Source: CAD feature listing. Evaluate the final solid. Frame: model axes, mm. Face numbers are marked on the shaded views. Round coordinates to 2 decimals unless told otherwise and drop trailing zeros. Loops run counter-clockwise (first coordinate to the right, second up) from the corner with the lowest first, then second, coordinate; pieces in that order, holes last. Notation, with made-up numbers: M 9.5,-19.5 L 21.5,-19.5 A25 ccw 21.5,18.5 Z; hole C 3,-31 d9. An arc over 180 degrees is marked long. Answer as CSV lines item,"result". Start each with the question number.
```python
from build123d import *

# Parameters (mm, degrees)
F0_R     = 15
F1_DEPTH = 180
F2_R     = 12.25
F3_DEPTH = 180
F4_R     = 12.25
F5_DEPTH = 180


# Not quite as in the source:
# - the program builds the solid bodies; features that only make, move or delete a surface that nothing else refers to are left out


with BuildPart() as f1:
    # F0 (on Front) → F1 (new body)
    with BuildSketch(Plane.XZ):
        Circle(F0_R)
    extrude(amount=F1_DEPTH)

    # F2 (on Front) → F3 (cut)
    with BuildSketch(Plane.XZ):
        Circle(F2_R)
    extrude(amount=-F3_DEPTH, mode=Mode.SUBTRACT)

    # F4 (on Front) → F5 (cut)
    with BuildSketch(Plane.XZ):
        Circle(F4_R)
    extrude(amount=F5_DEPTH, mode=Mode.SUBTRACT)


solid = f1.part
```
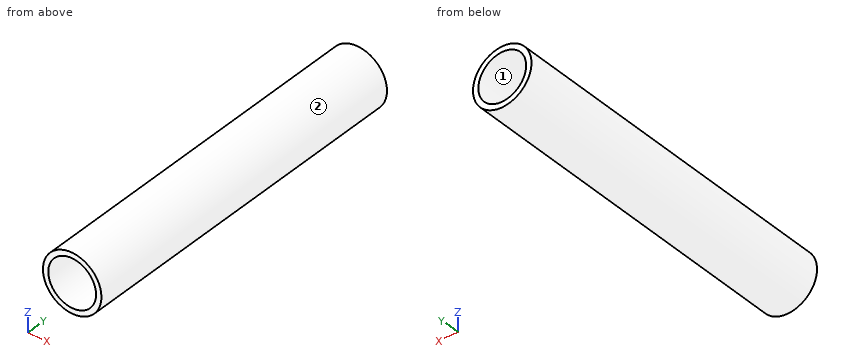
1) Ray query, line 1 along Z through (x, y) = (0, -47); line 2 along X through (y, z) = (-124, 0.75); line 3 along X through (y, z) = (-139, -7.5). Return the intervals inside material, ascending.
2) Section B-B, the plane x = 0. Return loops of the section in (y, z).
3) Section A-A, the plane z = 0. Return loops of the section in (x, y), and give its area (3 significant figures).
4) Mould query, pull axis Z, two halves, no side actions, for the marked faces 1 and 2. Classes: pulls with the +Z half, pulls with the -Z half, needs draft (parallel to the pull), parting line crosses it, or undercut.
5) Contact query for flat-ended pins moving along their axis: pin 1 Ø5 at (y, z) = (-108, -6) entering from -X; pin 2 Ø1 at (y, z) = (-84.5, 4) entering from +X; pin 3 Ø10 at (y, z) = (-30, 8) entering from -X. Output: stop coordinate, or through.
6) Section C-C, the plane y = -62. Return loops of the section in (x, z), and give its area (3 significant figures).
Findings below:
1,line 1,"-15 to -12.25, 12.25 to 15"
1,line 2,"-14.98 to -12.23, 12.23 to 14.98"
1,line 3,"-12.99 to -9.69, 9.69 to 12.99"
2,outline,"M -180,-15 L 0,-15 L 0,-12.25 L -180,-12.25 Z; M -180,12.25 L 0,12.25 L 0,15 L -180,15 Z"
3,outline,"M -15,-180 L -12.25,-180 L -12.25,0 L -15,0 Z; M 12.25,-180 L 15,-180 L 15,0 L 12.25,0 Z"
3,area,"990 mm²"
4,face 1,"undercut"
4,face 2,"parting line crosses it"
5,pin 1,"x = -14.59"
5,pin 2,"x = 14.59"
5,pin 3,"x = -14.7"
6,outline,"C 0,0 d30; hole C 0,0 d24.5"
6,area,"235 mm²"
